from build123d import *

# Parameters (mm, degrees)
SKETCH_R    = 35
PAD_DEPTH   = 8
SKETCH001_W = 20
SKETCH001_H = 3.7
SKETCH002_W = 20
SKETCH002_H = 3.2
FILLET_R    = 2


with BuildPart() as part:
    # Sketch → Pad (new body)
    with BuildSketch(Plane.XY):
        with BuildLine():
            ThreePointArc((-13.7, 40.759171), (0, -43), (13.7, 40.759171))
            Line((13.7, 45.5), (13.7, 40.759171))
            Line((-13.7, 45.5), (13.7, 45.5))
            Line((-13.7, 40.759171), (-13.7, 45.5))
        make_face()
        Circle(SKETCH_R, mode=Mode.SUBTRACT)
    extrude(amount=PAD_DEPTH)

    # Sketch001 → SubtractiveLoft section 0
    with BuildSketch(Plane.XY):
        with Locations((0, 40.25)):
            Rectangle(SKETCH001_W, SKETCH001_H)
    # Sketch002 (on Face7 of Pad) → SubtractiveLoft section 1
    with BuildSketch(Plane.XY.offset(8)):
        with Locations((0, 40.25)):
            Rectangle(SKETCH002_W, SKETCH002_H)
    loft(mode=Mode.SUBTRACT)

    # Fillet
    fillet_edges = [part.edges().sort_by_distance(p)[0] for p in [
        (-35, 0, 8),
        (0, -43, 8),
        (-13.7, 43.129585, 8),
        (13.7, 43.129585, 8),
        (-13.7, 45.5, 4),
        (13.7, 45.5, 4),
        (0, 45.5, 8),
    ]]
    fillet(fillet_edges, radius=FILLET_R)


solid = part.part
Verification items for the finished model (mm, model axes). A direction names the side the tool comes from. Give positions to 0.01 mm unless a question says otherwise; leave off trailing zeros. Use CSV: the item, a comma, the result in double quotes.
(1) Set-up check for faces 4 (the flat face through (13.7, 42, 3)), 5 (the cylindrical face through (-13.13, 41.89, 7.4)), 6 (the flat face through (0, 45.5, 3)), 7 (the flat face through (-13.7, 42, 3)), 8 (the cylindrical face through (13.13, 41.84, 7.4)): record each of +Z, -Z, +X, -X, +Y, -Y from which the full face is reachable in a straight line by a thin tool's end or side.
Derived:
face 4,"+Z, -Z, +X, +Y"
face 5,"+Z, -X, +Y"
face 6,"+Z, -Z, +X, -X, +Y"
face 7,"+Z, -Z, -X, +Y"
face 8,"+Z, +X, +Y"
(2) Sectioned sample at A-A (x = 0). Give the number of separate pieces and of enclosed holes in the cut face, plus the area to 3 significant figures.
Derived:
separate pieces,"3"
enclosed holes,"0"
area,"117 mm^2"
(3) Material ranges on L1, parallel to Y at x = 4, z = 7; L2, parallel to Y at x = -22, z = 5.25; L3, parallel to Y at x = -0.5, z = 1.25, recorded low to high.
Derived:
L1,"y = -42.54 to -35.04, 35.04 to 38.62, 41.88 to 45.23"
L2,"y = -36.95 to -27.22, 27.22 to 36.95"
L3,"y = -43 to -35, 35 to 38.44, 42.06 to 45.5"
(4) Go/stop test with flat-tipped pins: pin 1 (4 mm diameter, centred on y = 23, z = 7, fed in from +X); pin 2 (2 mm diameter, centred on x = -5, z = 1.5, fed in from -Y); pin 3 (3 mm diameter, centred on y = 42.5, z = 4, fed in from -X). Record where each tip stops, or that it passes through.
Derived:
pin 1,"stops at x = 37.43"
pin 2,"stops at y = -42.81"
pin 3,"stops at x = -13.7"
(5) Release check for a two-part mould opening along X. For faces 1 (the flat face through (-7, -35, 0)), 2 (the cylindrical face through (-13.13, 44.9, 3.04)), 3 (the cylindrical face through (-28, -21, 3)) record: +X half, -X half, draft (parallel to the pull), parting line (faces both ways), or undercut.
Derived:
face 1,"draft"
face 2,"-X half"
face 3,"undercut"
